Source: three-view drawing plus pictorial views. Frame: mm from the lowest corner of the part. Round coordinates to 2 decimals unless told otherwise and drop trailing zeros. Order: outer loops, then holes, each group sorted by start corner. A loop starts at its lowest first (then second) coordinate and runs counter-clockwise, first axis right, second up. Notation, with made-up numbers: (-31.5, 87) -> (-3.5, 87) arc R22 cw to (-3.5, 99) -> close; hole circle Ø10 at (17.25, 36.25). An arc over 180 degrees is marked (long way). Answer as CSV lines item,"result".
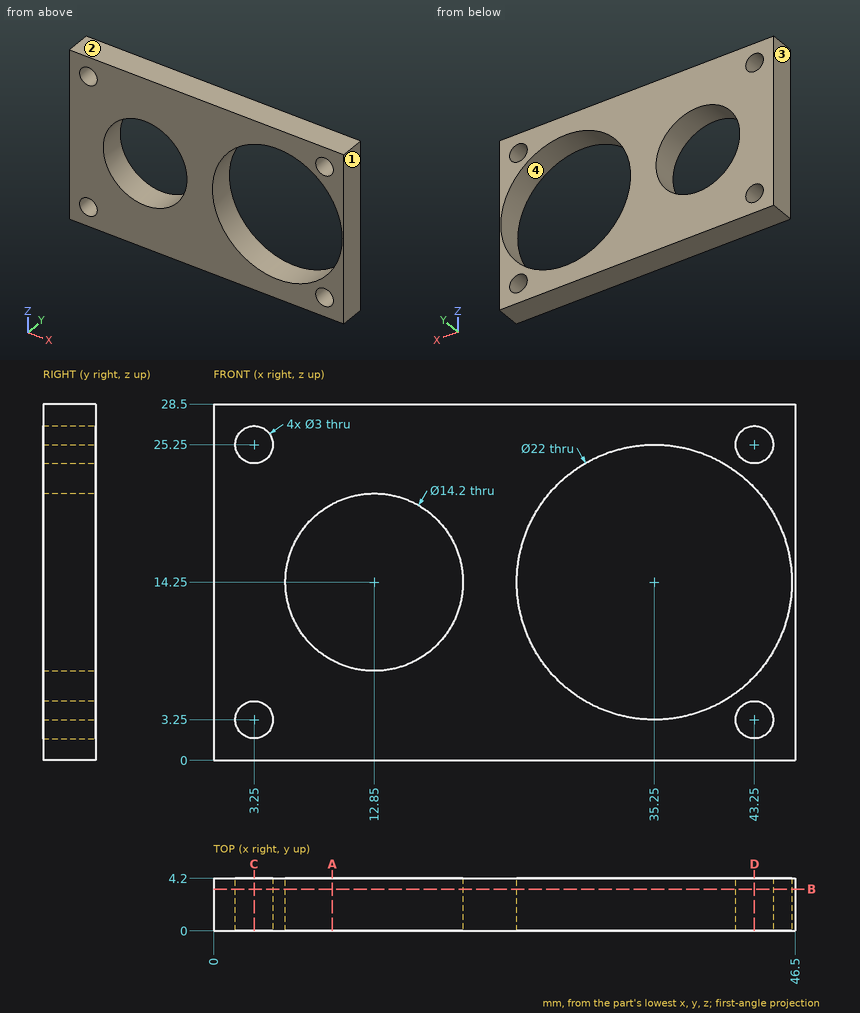
1. Section query B-B on y = 3.35. Return loops of the section in (x, z).
Results below:
outline,"(0, 0) -> (46.5, 0) -> (46.5, 28.5) -> (0, 28.5) -> close; hole circle Ø3 at (3.25, 3.25); hole circle Ø3 at (3.25, 25.25); hole circle Ø14.2 at (12.85, 14.25); hole circle Ø22 at (35.25, 14.25); hole circle Ø3 at (43.25, 3.25); hole circle Ø3 at (43.25, 25.25)"
2. Pin query (flat end, axial travel): pin 1 (1.8 mm diameter, centred on x = 43.25, z = 3.25, fed in from -Y). Return the tip coordinate at first contact, or that it passes through.
Results below:
pin 1,"through"
3. Line query: L1, parallel to Z at x = 3.25, y = 3.25; L2, parallel to X at y = 1.3, z = 14.5; L3, parallel to X at y = 3.7, z = 15.75. Output: solid intervals per line, ascending. Write a range as [from, to].
Results below:
L1,"[0, 1.75], [4.75, 23.75], [26.75, 28.5]"
L2,"[0, 5.75], [19.95, 24.25], [46.25, 46.5]"
L3,"[0, 5.91], [19.79, 24.35], [46.15, 46.5]"
4. Section query A-A on x = 9.5. Return loops of the section in (y, z).
Results below:
outline,"(0, 0) -> (4.2, 0) -> (4.2, 7.99) -> (0, 7.99) -> close; (0, 20.51) -> (4.2, 20.51) -> (4.2, 28.5) -> (0, 28.5) -> close"
5. Section query D-D on x = 43.25. Return loops of the section in (y, z), and give its area (3 significant figures).
Results below:
outline,"(0, 0) -> (4.2, 0) -> (4.2, 1.75) -> (0, 1.75) -> close; (0, 4.75) -> (4.2, 4.75) -> (4.2, 6.7) -> (0, 6.7) -> close; (0, 21.8) -> (4.2, 21.8) -> (4.2, 23.75) -> (0, 23.75) -> close; (0, 26.75) -> (4.2, 26.75) -> (4.2, 28.5) -> (0, 28.5) -> close"
area,"31.1 mm2"
6. Section query C-C on x = 3.25. Return loops of the section in (y, z), and give its area (3 significant figures).
Results below:
outline,"(0, 0) -> (4.2, 0) -> (4.2, 1.75) -> (0, 1.75) -> close; (0, 4.75) -> (4.2, 4.75) -> (4.2, 23.75) -> (0, 23.75) -> close; (0, 26.75) -> (4.2, 26.75) -> (4.2, 28.5) -> (0, 28.5) -> close"
area,"94.5 mm2"
7. Mould query, pull axis X, two halves, no side actions, for the marked faces 1, 2, 3 and 4. Classes: released by +X, released by -X, zero draft, split by the parting line, or undercut.
Results below:
face 1,"released by +X"
face 2,"zero draft"
face 3,"released by -X"
face 4,"undercut"
